Geometry: final body of the model. Coordinates: model frame, mm. A direction names the side the tool comes from. Give positions to 0.01 mm unless a question says otherwise; leave off trailing zeros. Write each loop counter-clockwise with the first axis right and the second up, starting at its lowest first coordinate (ties: lowest second). Pieces come first, ordered by that corner, then holes. Notation, with made-up numbers: (57.5, 76) -> (105.5, 76) arc R31 cw to (105.5, 111) -> close; hole circle Ø6 at (-3.75, -11). An arc over 180 degrees is marked (long way). Answer as a JSON object with one key per item and string values.
from build123d import *

# Parameters (mm, degrees)
F0_W         = 254
F0_H         = 53.975
F1_DEPTH     = 41.275
F3_DEPTH     = 22.225
F4_T1_DEPTH  = 38.1
F4_T3_DEPTH  = 37.5959026553
F6_DEPTH     = 11.43
F8_DEPTH     = 41.276
F9_T1_DEPTH  = 19.05
F9_T3_DEPTH  = 7.62
F10_W        = 37.30625
F10_H        = 41.275
F11_DEPTH    = 53.976
F12_W        = 19.05
F12_H        = 2.38125
F13_DEPTH    = 3.175
F14_T1_DEPTH = 15.5674179031


# Not quite as in the source:
# - a fillet or chamfer that OpenCascade refuses, or shapes differently, is made with other operations: its cross-section is extruded or revolved along the edge and cut away or added


with BuildPart() as f1:
    # F0 (on Top) → F1 (new body)
    with BuildSketch(Plane.XY):
        Rectangle(F0_W, F0_H)
    extrude(amount=F1_DEPTH)

    # F2 (on face) → F3 (cut)
    with BuildSketch(Plane.XY.offset(41.275)):
        Polygon((-80.16875, 16.66875), (-80.16875, -16.66875), (80.16875, -16.66875), (80.16875, -11.90625), (118.26875, -11.90625), (118.26875, 11.90625), (80.16875, 11.90625), (80.16875, 16.66875), align=None)
    extrude(amount=-F3_DEPTH, mode=Mode.SUBTRACT)

    # F4: fillet of radius 6.35 on 6 edges, made by hand

    # F4_s2 → F4_t1 (join)
    with BuildSketch(Plane.XY.offset(3.175)):
        with BuildLine():
            ThreePointArc((-80.16875, -10.31875), (-78.3088780605, -14.8088780605), (-73.81875, -16.66875))
            Line((-73.81875, -16.66875), (-80.16875, -16.66875))
            Line((-80.16875, -16.66875), (-80.16875, -10.31875))
        make_face()
        with BuildLine():
            ThreePointArc((111.91875, -11.90625), (116.4088780605, -10.0463780605), (118.26875, -5.55625))
            Line((118.26875, -5.55625), (118.26875, -11.90625))
            Line((118.26875, -11.90625), (111.91875, -11.90625))
        make_face()
        with BuildLine():
            ThreePointArc((118.26875, 5.55625), (116.4088780605, 10.0463780605), (111.91875, 11.90625))
            Line((111.91875, 11.90625), (118.26875, 11.90625))
            Line((118.26875, 11.90625), (118.26875, 5.55625))
        make_face()
        with BuildLine():
            ThreePointArc((-80.16875, 10.31875), (-78.3088780605, 14.8088780605), (-73.81875, 16.66875))
            Line((-73.81875, 16.66875), (-80.16875, 16.66875))
            Line((-80.16875, 16.66875), (-80.16875, 10.31875))
        make_face()
    extrude(amount=F4_T1_DEPTH)

    # F4_s4 → F4_t3 (join)
    with BuildSketch(Plane.XY.offset(3.6790973447)):
        with BuildLine():
            ThreePointArc((80.16875, 11.90625), (77.9089539046, 15.3388657855), (74.0203889379, 16.66875))
            Line((74.0203889379, 16.66875), (80.16875, 16.66875))
            Line((80.16875, 16.66875), (80.16875, 11.90625))
        make_face()
        with BuildLine():
            ThreePointArc((74.0203889379, -16.66875), (77.9089539046, -15.3388657855), (80.16875, -11.90625))
            Line((80.16875, -11.90625), (80.16875, -16.66875))
            Line((80.16875, -16.66875), (74.0203889379, -16.66875))
        make_face()
    extrude(amount=F4_T3_DEPTH)

    # F5 (on face) → F6 (cut)
    with BuildSketch(Plane(origin=(0, 0, 0), x_dir=(1, 0, 0), z_dir=(0, 0, -1))):
        with BuildLine():
            Line((-29.36875, 9.525), (-70.64375, 9.525))
            ThreePointArc((-70.64375, 9.525), (-80.16875, 0), (-70.64375, -9.525))
            Line((-70.64375, -9.525), (-29.36875, -9.525))
            Line((-29.36875, -9.525), (-29.36875, -11.90625))
            Line((-29.36875, -11.90625), (3.96875, -11.90625))
            Line((3.96875, -11.90625), (3.96875, -16.66875))
            Line((3.96875, -16.66875), (67.3851976236, -16.66875))
            Line((67.3851976236, -16.66875), (67.3851976236, 16.66875))
            Line((67.3851976236, 16.66875), (3.96875, 16.66875))
            Line((3.96875, 16.66875), (3.96875, 11.90625))
            Line((3.96875, 11.90625), (-29.36875, 11.90625))
            Line((-29.36875, 11.90625), (-29.36875, 9.525))
        make_face()
    extrude(amount=-F6_DEPTH, mode=Mode.SUBTRACT)

    # F7 (on face) → F8 (cut, through all)
    with BuildSketch(Plane(origin=(0, 0, 0), x_dir=(1, 0, 0), z_dir=(0, 0, -1))):
        with BuildLine():
            Line((-29.36875, 9.525), (-70.64375, 9.525))
            ThreePointArc((-70.64375, 9.525), (-72.2544463474, 9.3878262807), (-73.81875, 8.9802561211))
            Line((-73.81875, 8.9802561211), (-73.81875, -8.9802561211))
            ThreePointArc((-73.81875, -8.9802561211), (-72.2544463474, -9.3878262807), (-70.64375, -9.525))
            Line((-70.64375, -9.525), (-29.36875, -9.525))
            Line((-29.36875, -9.525), (-29.36875, -11.90625))
            Line((-29.36875, -11.90625), (3.96875, -11.90625))
            Line((3.96875, -11.90625), (3.96875, -16.66875))
            Line((3.96875, -16.66875), (67.3851976236, -16.66875))
            Line((67.3851976236, -16.66875), (67.3851976236, 16.66875))
            Line((67.3851976236, 16.66875), (3.96875, 16.66875))
            Line((3.96875, 16.66875), (3.96875, 11.90625))
            Line((3.96875, 11.90625), (-29.36875, 11.90625))
            Line((-29.36875, 11.90625), (-29.36875, 9.525))
        make_face()
    extrude(amount=-F8_DEPTH, mode=Mode.SUBTRACT)

    # F9: fillet of radius 6.35 on 8 edges, made by hand

    # F9_s2 → F9_t1 (join)
    with BuildSketch(Plane.XY):
        with BuildLine():
            ThreePointArc((3.96875, -11.90625), (6.2285460954, -15.3388657855), (10.1171110621, -16.66875))
            Line((10.1171110621, -16.66875), (3.96875, -16.66875))
            Line((3.96875, -16.66875), (3.96875, -11.90625))
        make_face()
        with BuildLine():
            ThreePointArc((-24.4117828388, -11.90625), (-27.1614134958, -11.2800626498), (-29.36875, -9.525))
            Line((-29.36875, -9.525), (-29.36875, -11.90625))
            Line((-29.36875, -11.90625), (-24.4117828388, -11.90625))
        make_face()
        with BuildLine():
            ThreePointArc((61.0351976236, -16.66875), (65.5253256842, -14.8088780605), (67.3851976236, -10.31875))
            Line((67.3851976236, -10.31875), (67.3851976236, -16.66875))
            Line((67.3851976236, -16.66875), (61.0351976236, -16.66875))
        make_face()
        with BuildLine():
            ThreePointArc((67.3851976236, 10.31875), (65.5253256842, 14.8088780605), (61.0351976236, 16.66875))
            Line((61.0351976236, 16.66875), (67.3851976236, 16.66875))
            Line((67.3851976236, 16.66875), (67.3851976236, 10.31875))
        make_face()
        with BuildLine():
            ThreePointArc((3.96875, 11.90625), (6.2285460954, 15.3388657855), (10.1171110621, 16.66875))
            Line((10.1171110621, 16.66875), (3.96875, 16.66875))
            Line((3.96875, 16.66875), (3.96875, 11.90625))
        make_face()
        with BuildLine():
            ThreePointArc((-29.36875, 9.525), (-27.1614134958, 11.2800626498), (-24.4117828388, 11.90625))
            Line((-24.4117828388, 11.90625), (-29.36875, 11.90625))
            Line((-29.36875, 11.90625), (-29.36875, 9.525))
        make_face()
    extrude(amount=F9_T1_DEPTH)

    # F9_s4 → F9_t3 (join)
    with BuildSketch(Plane.XY.offset(11.43)):
        with BuildLine():
            ThreePointArc((-73.81875, 3.175), (-71.9588780605, 7.6651280605), (-67.46875, 9.525))
            Line((-67.46875, 9.525), (-67.46875, 10.16))
            ThreePointArc((-67.46875, 10.16), (-70.64375, 10.16), (-74.0304166667, 9.5789398625))
            Line((-74.0304166667, 9.5789398625), (-74.45375, 8.9802561211))
            Line((-74.45375, 8.9802561211), (-74.45375, 3.175))
            Line((-74.45375, 3.175), (-73.81875, 3.175))
        make_face()
        with BuildLine():
            ThreePointArc((-73.81875, -3.175), (-71.9588780605, -7.6651280605), (-67.46875, -9.525))
            Line((-67.46875, -9.525), (-67.46875, -10.16))
            ThreePointArc((-67.46875, -10.16), (-70.64375, -10.16), (-74.0304166667, -9.5789398625))
            Line((-74.0304166667, -9.5789398625), (-74.45375, -8.9802561211))
            Line((-74.45375, -8.9802561211), (-74.45375, -3.175))
            Line((-74.45375, -3.175), (-73.81875, -3.175))
        make_face()
    extrude(amount=F9_T3_DEPTH)

    # F10 (on face) → F11 (cut, through all)
    with BuildSketch(Plane.XZ.offset(26.9875)):
        with Locations((-108.346875, 20.6375)):
            Rectangle(F10_W, F10_H)
    extrude(amount=-F11_DEPTH, mode=Mode.SUBTRACT)

    # F12 (on face) → F13 (cut)
    with BuildSketch(Plane.XY.offset(19.05)):
        with Locations((-31.75, 10.715625)):
            Rectangle(F12_W, F12_H)
        with Locations((-31.75, -10.715625)):
            Rectangle(F12_W, F12_H)
    extrude(amount=-F13_DEPTH, mode=Mode.SUBTRACT)

    # F14: fillet of radius 6.35 on 2 edges, made by hand

    # F14_s2 → F14_t1 (join)
    with BuildSketch(Plane.XY.offset(3.4825820969)):
        with BuildLine():
            ThreePointArc((-41.275, 9.525), (-39.0676634958, 11.2800626498), (-36.3180328388, 11.90625))
            Line((-36.3180328388, 11.90625), (-41.275, 11.90625))
            Line((-41.275, 11.90625), (-41.275, 9.525))
        make_face()
        with BuildLine():
            ThreePointArc((-36.3180328388, -11.90625), (-39.0676634958, -11.2800626498), (-41.275, -9.525))
            Line((-41.275, -9.525), (-41.275, -11.90625))
            Line((-41.275, -11.90625), (-36.3180328388, -11.90625))
        make_face()
    extrude(amount=F14_T1_DEPTH)


solid = f1.part
Q1. Cut plane B-B (x = 55.5). Return the cut outline in (y, z) (1 decimal).
Values:
{"outline": "(-27, 0) -> (-16.7, 0) -> (-16.7, 41.3) -> (-27, 41.3) -> close; (16.7, 0) -> (27, 0) -> (27, 41.3) -> (16.7, 41.3) -> close"}
Q2. Material intervals for L1, parallel to Y at x = 14, z = 20.5; L2, parallel to Y at x = 86.5, z = 39.5; L3, parallel to X at y = 5, z = 37, sorted ascending. Write a range as from..to.
Values:
{"L1": "-26.99..-16.67, 16.67..26.99", "L2": "-26.99..-11.91, 11.91..26.99", "L3": "-89.69..-80.17, 118.27..127"}
Q3. Set-up query: faces 4 (the cylindrical face through (-72.008, 7.615, 15.187)), 5 (the cylindrical face through (77.96, 15.3, 30.01)), 6 (the flat face through (127, 0, 20)). Return all of +Z, -Z, +X, -X, +Y, -Y with unobstructed straight access to the full face (end or side cutting, diameter ignored); none if empty.
Values:
{"face 4": "+Z, -Z", "face 5": "+Z", "face 6": "+Z, -Z, +X, +Y, -Y"}
Q4. First-contact query: P1, Ø1.5, axis at x = 45, y = 20.5, coming from the -Z side; P2, Ø2.5, axis at x = -30, y = 11, coming from the +Z side; P3, Ø4, axis at x = -56, y = 7, coming from the +Z side; P4, Ø16.5, axis at x = 87.5, y = 2, coming from the +Z side. Flat tips, straight axial feed; report the tip coordinate or a pass-through.
Values:
{"P1": "z = 0", "P2": "z = 19.05", "P3": "through", "P4": "z = 19.05"}
Q5. Cut plane A-A (z = 24). Return the cut outline in (x, y).
Values:
{"outline": "(-89.69, -26.99) -> (127, -26.99) -> (127, 26.99) -> (-89.69, 26.99) -> close; hole (-80.17, -10.32) arc R6.35 ccw to (-73.82, -16.67) -> (74.02, -16.67) arc R6.35 ccw to (80.17, -11.91) -> (111.92, -11.91) arc R6.35 ccw to (118.27, -5.56) -> (118.27, 5.56) arc R6.35 ccw to (111.92, 11.91) -> (80.17, 11.91) arc R6.35 ccw to (74.02, 16.67) -> (-73.82, 16.67) arc R6.35 ccw to (-80.17, 10.32) -> close"}
Q6. Cut plane D-D (y = 14). Return the cut outline in (x, z) (3 decimals), and give its area (3 significant figures).
Values:
{"outline": "(-89.694, 0) -> (4.943, 0) -> (4.943, 19.05) -> (-78.993, 19.05) -> (-78.993, 41.275) -> (-89.694, 41.275) -> close; (66.209, 0) -> (127, 0) -> (127, 41.275) -> (79.194, 41.275) -> (79.194, 19.05) -> (66.209, 19.05) -> close", "area": "4,260 mm²"}
Q7. Mould query, pull axis X, two halves, no side actions, for faces 1 (the cylindrical face through (116.359, -10.095, 30.007)), 2 (the flat face through (20, 18, 0)), 3 (the flat face through (-89.694, 0, 20)). Classes: pulls with the +X half, pulls with the -X half, needs draft (parallel to the pull), parting line crosses it, or undercut.
Values:
{"face 1": "undercut", "face 2": "needs draft", "face 3": "pulls with the -X half"}
